Can you work these out from the drawing? Everything is in mm from the part's minimum corner. Coordinates: 2 decimals unless noted, no trailing zeros. Loops run counter-clockwise (first coordinate to the right, second up) from the corner with the lowest first, then second, coordinate; pieces in that order, holes last. Notation, with made-up numbers: (-34.5, -6.5) - (16.5, -6.5) arc R15 ccw to (16.5, 1.5) - close; hole circle Ø1 at (-9, 79). An arc over 180 degrees is marked (long way). Put each result on its own line as item: value. Start each with the question number.
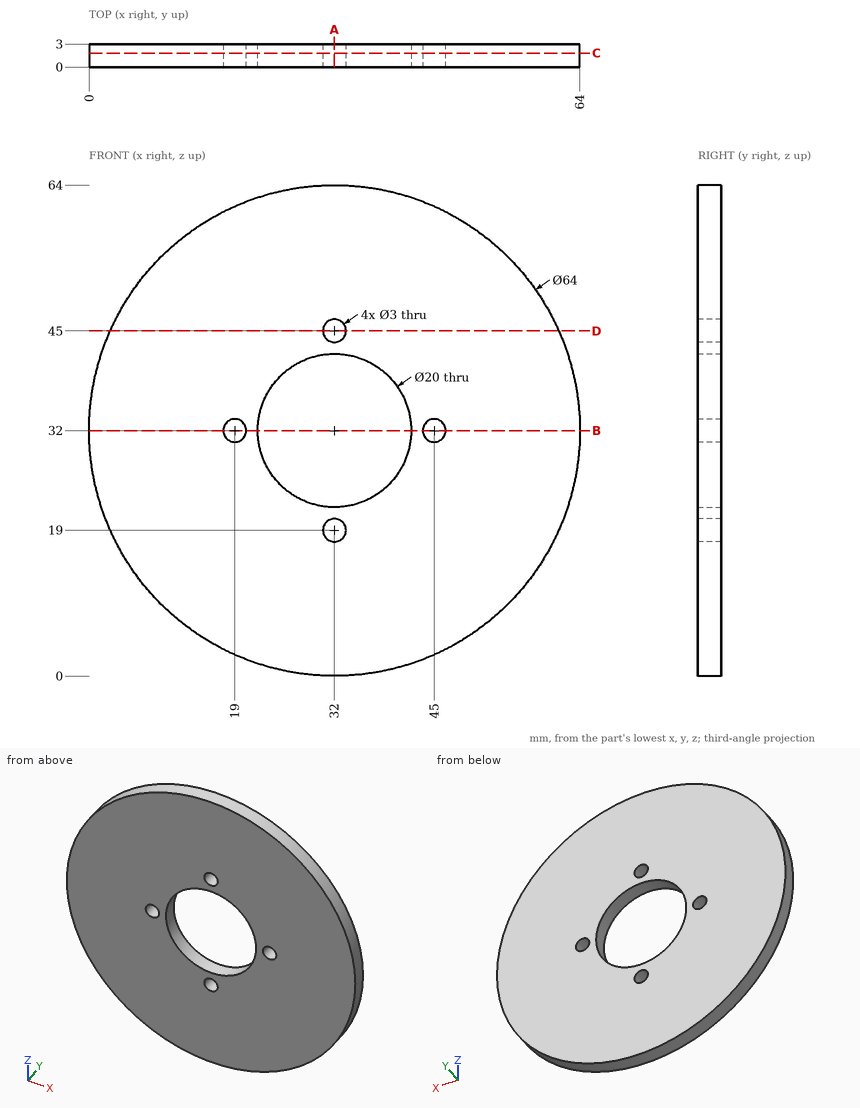
(1) For pin 1 Ø1.5 at (y, z) = (2, 35) entering from -X; pin 2 Ø3 at (x, z) = (21.5, 47) entering from -Y; pin 3 Ø2.5 at (x, z) = (45, 32) entering from +Y; pin 4 Ø1 at (x, y) = (23, 2.5) entering from -Z, each with a flat end and sliding along its axis, tell me the tip position at first contact or that it passes through.
(2) I want a section at A-A on x = 32. List the corners of the cut face in (y, z) for me, and give its area (3 significant figures).
(3) I want a section at D-D on z = 45. List the corners of the cut face in (x, y) for me.
(4) I want a section at B-B on z = 32. List the corners of the cut face in (x, y) for me.
(5) I want a section at C-C on y = 1.8. List the corners of the cut face in (x, z) for me, and give its area (3 significant figures).
(6) I need wall thicknesses on L1, parallel to Z at x = 32, y = 0.6; L2, parallel to X at y = 1.65, z = 34.5; L3, parallel to X at y = 0.9, z = 20. Which ranges of each line are inside material? Lowest first, please. Write a range as [from, to].
Answer sheet:
1. pin 1: stops at x = 0.08
1. pin 2: stops at y = 0
1. pin 3: passes through
1. pin 4: stops at z = 1.15
2. outline: (0, 0) - (3, 0) - (3, 17.5) - (0, 17.5) - close; (0, 20.5) - (3, 20.5) - (3, 22) - (0, 22) - close; (0, 42) - (3, 42) - (3, 43.5) - (0, 43.5) - close; (0, 46.5) - (3, 46.5) - (3, 64) - (0, 64) - close
2. area: 114 mm^2
3. outline: (2.76, 0) - (30.5, 0) - (30.5, 3) - (2.76, 3) - close; (33.5, 0) - (61.24, 0) - (61.24, 3) - (33.5, 3) - close
4. outline: (0, 0) - (17.5, 0) - (17.5, 3) - (0, 3) - close; (20.5, 0) - (22, 0) - (22, 3) - (20.5, 3) - close; (42, 0) - (43.5, 0) - (43.5, 3) - (42, 3) - close; (46.5, 0) - (64, 0) - (64, 3) - (46.5, 3) - close
5. outline: circle Ø64 at (32, 32); hole circle Ø3 at (19, 32); hole circle Ø20 at (32, 32); hole circle Ø3 at (32, 19); hole circle Ø3 at (32, 45); hole circle Ø3 at (45, 32)
5. area: 2,870 mm^2
6. L1: z = [0, 17.5], [20.5, 22], [42, 43.5], [46.5, 64]
6. L2: x = [0.1, 22.32], [41.68, 63.9]
6. L3: x = [2.34, 30.88], [33.12, 61.66]
